from build123d import *

# Parameters (mm, degrees)
F0_W     = 152.2748842835
F0_H     = 37.9443131387
F1_DEPTH = 5
F5_R     = 0.6498911682
F6_DEPTH = 37.9
F2_W     = 152.2748842835
F2_H     = 1.4094897779
F2_H_2   = 1.7610266805
F7_DEPTH = 6


# Not quite as in the source:
# - the program builds the solid bodies; features that only make, move or delete a surface that nothing else refers to are left out


with BuildPart() as f1:
    # F0 (on Top) → F1 (new body)
    with BuildSketch(Plane.XY):
        with Locations((0.995259732, -18.9721565694)):
            Rectangle(F0_W, F0_H)
    extrude(amount=F1_DEPTH)

    # F5 (on Front) → F6 (join)
    with BuildSketch(Plane.XZ):
        with Locations((-59.8872974515, 5.076338537)):
            Circle(F5_R)
        with Locations((-56.5108135343, 4.9978159368)):
            Circle(F5_R)
        with Locations((-46.1065284908, 4.9978159368)):
            Circle(F5_R)
        with Locations((-49.9934107065, 4.958554171)):
            Circle(F5_R)
        with Locations((-53.3306375146, 5.0370772369)):
            Circle(F5_R)
        with Locations((-30.849635601, 5.0810105167)):
            Circle(F5_R)
        with Locations((-14.1990464181, 5.1284483634)):
            Circle(F5_R)
        with Locations((-17.1876139939, 5.0810105167)):
            Circle(F5_R)
        with Locations((-20.650556311, 5.0810105167)):
            Circle(F5_R)
        with Locations((-24.3506878614, 5.0810105167)):
            Circle(F5_R)
        with Locations((-27.6713185012, 5.0335731357)):
            Circle(F5_R)
        with Locations((1.6279553529, 5.0831306726)):
            Circle(F5_R)
        with Locations((19.4284114987, 5.2831359208)):
            Circle(F5_R)
        with Locations((16.2283293903, 5.1497989334)):
            Circle(F5_R)
        with Locations((13.2282525301, 5.0831306726)):
            Circle(F5_R)
        with Locations((9.361486882, 5.0164619461)):
            Circle(F5_R)
        with Locations((5.4947216995, 5.0164619461)):
            Circle(F5_R)
        with Locations((49.0938574076, 5.0953882746)):
            Circle(F5_R)
        with Locations((45.4649962485, 5.1608970389)):
            Circle(F5_R)
        with Locations((42.1599261463, 5.0851320848)):
            Circle(F5_R)
        with Locations((38.728825748, 4.870061297)):
            Circle(F5_R)
        with Locations((35.5742499232, 4.9827247858)):
            Circle(F5_R)
    extrude(amount=F6_DEPTH)

    # F2 (on face) → F7 (join)
    with BuildSketch(Plane.XY.offset(5)):
        with Locations((0.995259732, -0.7047448889)):
            Rectangle(F2_W, F2_H)
        with Locations((0.995259732, -37.0637997985)):
            Rectangle(F2_W, F2_H_2)
    extrude(amount=F7_DEPTH)


solid = f1.part
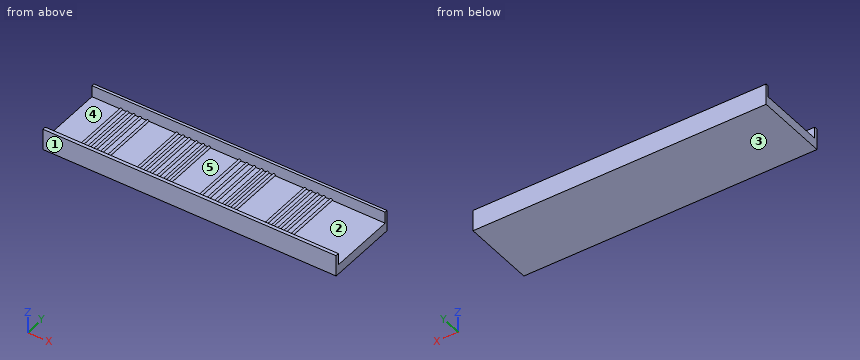
Part model, mm, in its own coordinate system. Face numbers are marked on the shaded views. A direction names the side the tool comes from. Round coordinates to 2 decimals unless told otherwise and drop trailing zeros. Write each loop counter-clockwise with the first axis right and the second up, starting at its lowest first coordinate (ties: lowest second). Pieces come first, ordered by that corner, then holes. Notation, with made-up numbers: M 86.5,6 L 104.5,6 A11 cw 104.5,10 Z; hole C 45,-11 d2. An arc over 180 degrees is marked long. Return JSON: item names as keys, results as strings. Group by question number.
(1) Pin check, flat tips, straight feed: pin 1 Ø1.7 at (x, y) = (41, -21) entering from +Z; pin 2 Ø1.4 at (x, y) = (-16, -15.5) entering from +Z; pin 3 Ø1 at (x, y) = (25.5, -25.5) entering from +Z. Stop position of each tip, or through.
(2) Drill centre lines: probe 1 along Y at (x, z) = (13.5, 6.5); probe 2 along Z at (x, y) = (-48.5, -27.5); probe 3 along Z at (x, y) = (42.5, -29). Where is each one in solid material? Low to high.
(3) Saw through at B-B on x = 58. Write the cut outline in (y, z), then the cut area to 3 significant figures.
(4) Saw through at A-A on z = 8.25. Write the cut outline in (x, y).
(5) Which spindle directions (+Z, -Z, +X, -X, +Y, -Y) get a long thin tool onto all of the face, cutting with end or side? Do the marked faces 1, 2, 3, 4 and 5. Say none if no direction does.
Returned:
{
 "1": {"pin 1": "z = 5.66", "pin 2": "z = 5.51", "pin 3": "z = 5"},
 "2": {"probe 1": "-37.94 to -36.18, -1.41 to 0", "probe 2": "0 to 5", "probe 3": "0 to 5.64"},
 "3": {"outline": "M -37.94,0 L 0,0 L 0,11 L -1.41,11 L -1.41,5 L -36.18,5 L -36.18,11 L -37.94,11 Z", "area": "209 mm²"},
 "4": {"outline": "M -75.14,-37.94 L 77.13,-37.94 L 77.13,-36.18 L -75.14,-36.18 Z; M -75.14,-1.41 L 77.13,-1.41 L 77.13,0 L -75.14,0 Z"},
 "5": {"face 1": "+Z, -Z, +X, -X, -Y", "face 2": "+Z, +X", "face 3": "-Z, +X, -X, +Y, -Y", "face 4": "+Z, -X", "face 5": "+Z"}
}
